Verification items for the finished model (mm, model axes). Face numbers are marked on the shaded views. A direction names the side the tool comes from. Round coordinates to 2 decimals unless told otherwise and drop trailing zeros. Order: outer loops, then holes, each group sorted by start corner. A loop starts at its lowest first (then second) coordinate and runs counter-clockwise, first axis right, second up. Notation, with made-up numbers: (15, -35.75) -> (56, -35.75) arc R16 ccw to (56, -5.75) -> close; hole circle Ø1 at (41, 11.5). An arc over 180 degrees is marked (long way). Return JSON: item names as keys, results as strings. Group by question number.
1) Section check C-C on y = 2.25. Enter the section's corners in (x, z), plus the area to 3 significant figures.
2) Depth check by flat-ended pin: pin 1 (0.6 mm diameter, centred on x = -0.5, z = 3.5, fed in from +Y); pin 2 (1.5 mm diameter, centred on x = 0.5, y = 13, fed in from +Z). Enter the tip coordinate at first touch or a pass-through.
3) Section check A-A on x = 0.95. Enter the section's corners in (y, z), plus the area to 3 significant figures.
4) Tool access check on the marked faces 4, 5 and 6. Record the directions out of +Z, -Z, +X, -X, +Y, -Y that give a thin tool (end or side, any length) a straight path to the whole face; none if there is none.
5) Section check D-D on y = 22.75. Enter the section's corners in (x, z), plus the area to 3 significant figures.
6) Section check B-B on z = -2.25. Enter the section's corners in (x, y), plus the area to 3 significant figures.
7) Scan lines: L1, parallel to Z at x = 0.65, y = 21.25; L2, parallel to Y at x = 1.35, z = 2; L3, parallel to Z at x = -0.05, y = 24.75. Record each from-to range of solid material in increasing order.
8) Draft check along Y on the marked faces 1, 2 and 3. Enter one of: pulls with the +Y half, pulls with the -Y half, needs draft (parallel to the pull), parting line crosses it, or undercut.
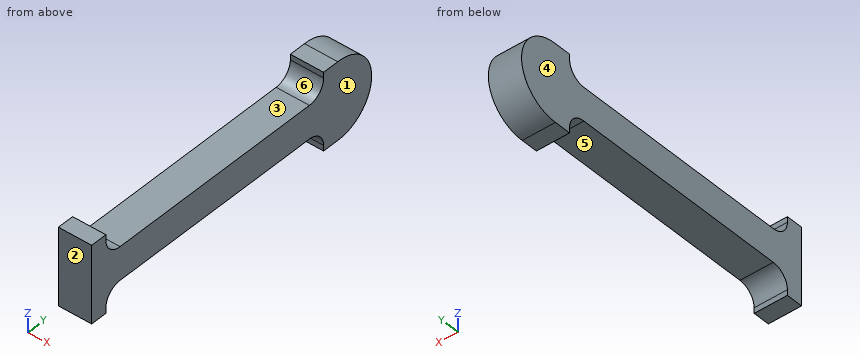
```python
from build123d import *

# Parameters (mm, degrees)
SKETCH1_W           = 3
SKETCH1_H           = 3
BOSS_EXTRUDE1_DEPTH = 23
SKETCH3_W           = 3
SKETCH3_H           = 7
BOSS_EXTRUDE2_DEPTH = 1.5
FILLET1_R           = 1.5
BOSS_EXTRUDE3_DEPTH = 3


with BuildPart() as part:
    # Sketch1 → Boss-Extrude1 (new body)
    with BuildSketch(Plane(origin=(0, 0, 0), x_dir=(1, 0, 0), z_dir=(0, 1, 0))):
        Rectangle(SKETCH1_W, SKETCH1_H)
    extrude(amount=BOSS_EXTRUDE1_DEPTH)

    # Sketch3 → Boss-Extrude2 (add)
    with BuildSketch(Plane(origin=(0, 23, 0), x_dir=(1, 0, 0), z_dir=(0, 1, 0))):
        Rectangle(SKETCH3_W, SKETCH3_H)
    boss_extrude2 = extrude(amount=BOSS_EXTRUDE2_DEPTH)

    # Mirror2: Boss-Extrude2 across plane
    add(boss_extrude2.mirror(Plane(origin=(0, 11.5, 0), x_dir=(0, 0, 1), z_dir=(0, -1, 0))))

    # Fillet1
    fillet1_edges = [part.edges().sort_by_distance(p)[0] for p in [
        (0, 23, 1.5),
        (0, 0, 1.5),
        (0, 0, -1.5),
        (0, 23, -1.5),
    ]]
    fillet(fillet1_edges, radius=FILLET1_R)

    # Sketch4 → Boss-Extrude3 (add)
    with BuildSketch(Plane.ZY.offset(1.5)):
        with BuildLine():
            Line((-3.5, 24.5), (3.5, 24.5))
            ThreePointArc((3.5, 24.5), (0, 28.077563248), (-3.5, 24.5))
        make_face()
    extrude(amount=-BOSS_EXTRUDE3_DEPTH)


solid = part.part
```
Check result:
{
 "1": {"outline": "(-1.5, -1.5) -> (1.5, -1.5) -> (1.5, 1.5) -> (-1.5, 1.5) -> close", "area": "9.00 mm^2"},
 "2": {"pin 1": "y = 26", "pin 2": "z = 1.5"},
 "3": {"outline": "(-1.5, -3.5) -> (0, -3.5) -> (0, -3) arc R1.5 cw to (1.5, -1.5) -> (21.5, -1.5) arc R1.5 cw to (23, -3) -> (23, -3.5) -> (24.5, -3.5) arc R3.5 ccw (long way) to (24.5, 3.5) -> (23, 3.5) -> (23, 3) arc R1.5 cw to (21.5, 1.5) -> (1.5, 1.5) arc R1.5 cw to (0, 3) -> (0, 3.5) -> (-1.5, 3.5) -> close", "area": "112 mm^2"},
 "4": {"face 4": "+Z, -Z, -X, +Y, -Y", "face 5": "-Z, +X, -X", "face 6": "+Z, +X, -X"},
 "5": {"outline": "(-1.5, -2.17) -> (1.5, -2.17) -> (1.5, 2.17) -> (-1.5, 2.17) -> close", "area": "13.0 mm^2"},
 "6": {"outline": "(-1.5, -1.5) -> (1.5, -1.5) -> (1.5, 0.2) -> (-1.5, 0.2) -> close; (-1.5, 22.8) -> (1.5, 22.8) -> (1.5, 27.26) -> (-1.5, 27.26) -> close", "area": "18.5 mm^2"},
 "7": {"L1": "-1.5 to 1.5", "L2": "-1.5 to 0.38, 22.62 to 27.45", "L3": "-3.5 to 3.5"},
 "8": {"face 1": "needs draft", "face 2": "pulls with the -Y half", "face 3": "undercut"}
}
